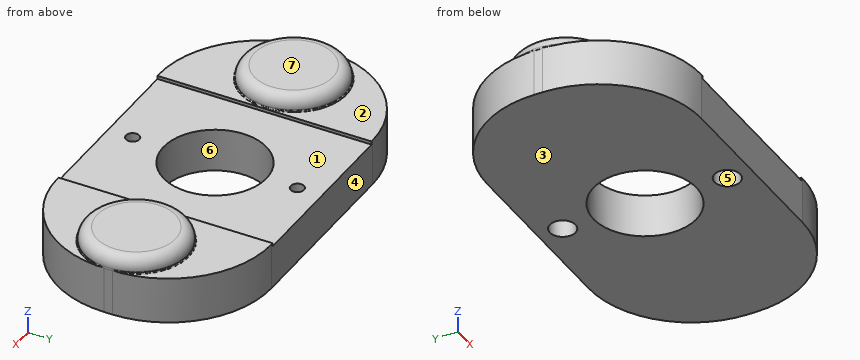
```python
from build123d import *

# Parameters (mm, degrees)
F0_R          = 1.625
F1_DEPTH      = 11.3
F2_R          = 12.5
F3_DEPTH      = 11.301
F4_R          = 9.5
F5_DEPTH      = 10.5
F6_R          = 3.125
F7_DEPTH      = 5
F8_W          = 44
F8_H          = 52
F9_DEPTH      = 0.8
F10_R         = 12.539936204
F10_R_2       = 9.5
F11_DEPTH     = 1
F12_R         = 12.54
F13_DEPTH     = 2.5
F16_T4_ANGLE  = 178.2861059353
F16_S5_R      = 25
F16_T6_DEPTH  = 17
F16_T10_ANGLE = 178.2861059353
F16_S11_R     = 25
F16_T12_DEPTH = 17
F16_T16_ANGLE = 356.5984947452
F16_S17_R     = 25
F16_T18_DEPTH = 21
F16_T22_ANGLE = 356.5984947452
F16_S23_R     = 25
F16_T24_DEPTH = 21


# Not quite as in the source:
# - a fillet or chamfer that OpenCascade refuses, or shapes differently, is made with other operations: its cross-section is extruded or revolved along the edge and cut away or added
# - a feature of the source that left no trace in its solid (it failed there, or was rolled back) is left out


with BuildPart() as f1:
    # F0 (on Top) → F1 (new body)
    with BuildSketch(Plane.XY):
        with BuildLine():
            Line((-22.5, -26), (22.5, -26))
            ThreePointArc((22.5, -26), (40.1776695297, -18.6776695297), (47.5, -1))
            Line((47.5, -1), (47.5, 1))
            ThreePointArc((47.5, 1), (40.1776695297, 18.6776695297), (22.5, 26))
            Line((22.5, 26), (-22.5, 26))
            ThreePointArc((-22.5, 26), (-40.1776695297, 18.6776695297), (-47.5, 1))
            Line((-47.5, 1), (-47.5, -1))
            ThreePointArc((-47.5, -1), (-40.1776695297, -18.6776695297), (-22.5, -26))
        make_face()
        with Locations((0, -20)):
            Circle(F0_R, mode=Mode.SUBTRACT)
        with Locations((0, 20)):
            Circle(F0_R, mode=Mode.SUBTRACT)
    extrude(amount=F1_DEPTH)

    # F2 (on face) → F3 (cut, through all)
    with BuildSketch(Plane(origin=(0, 0, 0), x_dir=(1, 0, 0), z_dir=(0, 0, -1))):
        Circle(F2_R)
    extrude(amount=-F3_DEPTH, mode=Mode.SUBTRACT)

    # F4 (on face) → F5 (cut)
    with BuildSketch(Plane.XY.offset(11.3)):
        with Locations((-35, 0)):
            Circle(F4_R)
        with Locations((35, 0)):
            Circle(F4_R)
    extrude(amount=-F5_DEPTH, mode=Mode.SUBTRACT)

    # F6 (on face) → F7 (cut)
    with BuildSketch(Plane(origin=(0, 0, 0), x_dir=(1, 0, 0), z_dir=(0, 0, -1))):
        with Locations((0, 20)):
            Circle(F6_R)
        with Locations((0, -20)):
            Circle(F6_R)
    extrude(amount=-F7_DEPTH, mode=Mode.SUBTRACT)

    # F8 (on face) → F9 (cut)
    with BuildSketch(Plane.XY.offset(11.3)):
        Rectangle(F8_W, F8_H)
    extrude(amount=-F9_DEPTH, mode=Mode.SUBTRACT)

    # F10 (on face) → F11 (join)
    with BuildSketch(Plane.XY.offset(11.3)):
        with Locations((-35, 0)):
            Circle(F10_R)
        with Locations((-35, 0)):
            Circle(F10_R_2, mode=Mode.SUBTRACT)
        with Locations((35, 0)):
            Circle(F10_R)
        with Locations((35, 0)):
            Circle(F10_R_2, mode=Mode.SUBTRACT)
    extrude(amount=F11_DEPTH)

    # F12 (on face) → F13 (join)
    with BuildSketch(Plane.XY.offset(12.3)):
        with Locations((-35, 0)):
            Circle(F12_R)
        with Locations((35, 0)):
            Circle(F12_R)
    extrude(amount=F13_DEPTH)

    # F14: fillet of radius 3 on 1 edges, made by hand

    # F14_s1 → F14_t2 (revolve, cut)
    with BuildSketch(Plane.XZ):
        with BuildLine():
            ThreePointArc((-22.46, 11.8), (-23.3386796564, 13.9213203436), (-25.46, 14.8))
            Line((-25.46, 14.8), (-22.46, 14.8))
            Line((-22.46, 14.8), (-22.46, 11.8))
        make_face()
    revolve(axis=Axis((-35, 0, 14.8), (0, 0, 1)), mode=Mode.SUBTRACT)

    # F15: fillet of radius 3 on 1 edges, made by hand

    # F15_s1 → F15_t2 (revolve, cut)
    with BuildSketch(Plane.XZ):
        with BuildLine():
            ThreePointArc((47.54, 11.8), (46.6613203436, 13.9213203436), (44.54, 14.8))
            Line((44.54, 14.8), (47.54, 14.8))
            Line((47.54, 14.8), (47.54, 11.8))
        make_face()
    revolve(axis=Axis((35, 0, 14.8), (0, 0, 1)), mode=Mode.SUBTRACT)

    # F16: fillet of radius 0.25 on 3 edges, made by hand


with BuildPart() as f16_tool2:
    # F16_s3 → F16_t4 (revolve)
    with BuildSketch(Plane.XZ):
        with BuildLine():
            ThreePointArc((-22.460063796, 11.55), (-22.3868404913, 11.3732233047), (-22.210063796, 11.3))
            Line((-22.210063796, 11.3), (-22.460063796, 11.3))
            Line((-22.460063796, 11.3), (-22.460063796, 11.55))
        make_face()
    revolve(axis=Axis((-35, 0, 11.3), (0, 0, 1)), revolution_arc=F16_T4_ANGLE)

    # F16_s5 → F16_t6 (intersect, symmetric)
    with BuildSketch(Plane.XY.offset(11.5)):
        with Locations((-22.5, 1)):
            Circle(F16_S5_R)
    extrude(amount=F16_T6_DEPTH, both=True, mode=Mode.INTERSECT)


with BuildPart() as f1_1:
    add(f1.part)

    # F16_t1: union F16_tool2
    add(f16_tool2.part)


with BuildPart() as f16_tool8:
    # F16_s9 → F16_t10 (revolve)
    with BuildSketch(Plane(origin=(-0.0313084228, 1.046333877, 0), x_dir=(0, 0, 1), z_dir=(-0.0299086337, 0.9995526367, 0))):
        with BuildLine():
            ThreePointArc((11.55, -47.5242784902), (11.3732233047, -47.5975017949), (11.3, -47.7742784902))
            Line((11.3, -47.7742784902), (11.3, -47.5242784902))
            Line((11.3, -47.5242784902), (11.55, -47.5242784902))
        make_face()
    revolve(axis=Axis((-35, 0, 11.3), (0, 0, 1)), revolution_arc=F16_T10_ANGLE)

    # F16_s11 → F16_t12 (intersect, symmetric)
    with BuildSketch(Plane.XY.offset(11.5)):
        with Locations((-22.5, -1)):
            Circle(F16_S11_R)
    extrude(amount=F16_T12_DEPTH, both=True, mode=Mode.INTERSECT)


with BuildPart() as f1_2:
    add(f1_1.part)

    # F16_t7: union F16_tool8
    add(f16_tool8.part)


with BuildPart() as f16_tool14:
    # F16_s15 → F16_t16 (revolve)
    with BuildSketch(Plane(origin=(0.0308302837, -1.0383204819, 0), x_dir=(0, 0, 1), z_dir=(0.0296793741, -0.9995594703, 0))):
        with BuildLine():
            ThreePointArc((11.55, -47.524517666), (11.3732233047, -47.5977409707), (11.3, -47.774517666))
            Line((11.3, -47.774517666), (11.3, -47.524517666))
            Line((11.3, -47.524517666), (11.55, -47.524517666))
        make_face()
    revolve(axis=Axis((35, 0, 11.3), (0, 0, 1)), revolution_arc=F16_T16_ANGLE)

    # F16_s17 → F16_t18 (intersect, symmetric)
    with BuildSketch(Plane.XY.offset(11.5)):
        with Locations((22.5, 1)):
            Circle(F16_S17_R)
    extrude(amount=F16_T18_DEPTH, both=True, mode=Mode.INTERSECT)


with BuildPart() as f1_3:
    add(f1_2.part)

    # F16_t13: union F16_tool14
    add(f16_tool14.part)


with BuildPart() as f16_tool20:
    # F16_s21 → F16_t22 (revolve)
    with BuildSketch(Plane(origin=(0.0308302837, -1.0383204819, 0), x_dir=(0, 0, 1), z_dir=(0.0296793741, -0.9995594703, 0))):
        with BuildLine():
            ThreePointArc((11.55, -47.524517666), (11.3732233047, -47.5977409707), (11.3, -47.774517666))
            Line((11.3, -47.774517666), (11.3, -47.524517666))
            Line((11.3, -47.524517666), (11.55, -47.524517666))
        make_face()
    revolve(axis=Axis((35, 0, 11.3), (0, 0, 1)), revolution_arc=F16_T22_ANGLE)

    # F16_s23 → F16_t24 (intersect, symmetric)
    with BuildSketch(Plane.XY.offset(11.5)):
        with Locations((22.5, -1)):
            Circle(F16_S23_R)
    extrude(amount=F16_T24_DEPTH, both=True, mode=Mode.INTERSECT)


with BuildPart() as f1_4:
    add(f1_3.part)

    # F16_t19: union F16_tool20
    add(f16_tool20.part)


solid = f1_4.part
```
Verification items for the finished model (mm, model axes). Face numbers are marked on the shaded views. A direction names the side the tool comes from. Give positions to 0.01 mm unless a question says otherwise; leave off trailing zeros. Order: outer loops, then holes, each group sorted by start corner. A loop starts at its lowest first (then second) coordinate and runs counter-clockwise, first axis right, second up. Notation, with made-up numbers: M 56,-23 L 106,-23 A15 ccw 106,-16 Z; hole C 49.25,39.25 d5. An arc over 180 degrees is marked long. Answer in a Markdown table with one row per item. Add a question column.
Item 1: Gauge pin test, flat ends, axial feed: pin 1 (0.6 mm diameter, centred on y = -0.5, z = 6.5, fed in from +X); pin 2 (10 mm diameter, centred on x = 8, y = 18.5, fed in from +Z); pin 3 (6 mm diameter, centred on y = 10.5, z = 6, fed in from +X); pin 4 (2.5 mm diameter, centred on x = 0, y = 20, fed in from -Z). Record the tip position at first contact, or that the pin passes through.
Item 2: Section check A-A, the plane x = 0. Enter the section's corners in (y, z) (3 decimals), and give its area (3 significant figures).
Item 3: Section check C-C, the plane x = -11.5. Enter the section's corners in (y, z).
Item 4: Mould release check, pull along X, two halves, no side actions. Record for the marked faces 6 and 7: released by +X, released by -X, zero draft, split by the parting line, or undercut.
Item 5: Scan lines: probe 1 along Y at (x, z) = (0, 3.2) (3 decimals); probe 2 along Z at (x, y) = (33, -3); probe 3 along X at (y, z) = (6.5, 7.5). Record each from-to range of solid material in increasing order. Write a range as from..to.
Item 6: Section check D-D, the plane y = 20. Enter the section's corners in (x, z) (3 decimals).
Item 7: Section check B-B, the plane z = 9.5. Enter the section's corners in (x, y) (3 decimals).
Item 8: Tool access check on the marked faces 1, 2, 3, 4 and 5. Record the directions out of +Z, -Z, +X, -X, +Y, -Y that give a thin tool (end or side, any length) a straight path to the whole face; none if there is none.
Filled sheet:
| question | item | result |
|---|---|---|
| 1 | pin 1 | stops at x = 47.5 |
| 1 | pin 2 | stops at z = 10.5 |
| 1 | pin 3 | stops at x = 46.64 |
| 1 | pin 4 | passes through |
| 2 | outline | M -26,0 L -23.125,0 L -23.125,5 L -21.625,5 L -21.625,10.5 L -26,10.5 Z; M -18.375,5 L -16.875,5 L -16.875,0 L -12.5,0 L -12.5,10.5 L -18.375,10.5 Z; M 12.5,0 L 16.875,0 L 16.875,5 L 18.375,5 L 18.375,10.5 L 12.5,10.5 Z; M 21.625,5 L 23.125,5 L 23.125,0 L 26,0 L 26,10.5 L 21.625,10.5 Z |
| 2 | area | 185 mm^2 |
| 3 | outline | M -26,0 L -4.9,0 L -4.9,10.5 L -26,10.5 Z; M 4.9,0 L 26,0 L 26,10.5 L 4.9,10.5 Z |
| 4 | face 6 | undercut |
| 4 | face 7 | zero draft |
| 5 | probe 1 | y = -26..-23.125, -16.875..-12.5, 12.5..16.875, 23.125..26 |
| 5 | probe 2 | z = 0..0.8, 12.3..14.8 |
| 5 | probe 3 | x = -46.89..-41.93, -28.07..-10.68, 10.68..28.07, 41.93..46.89 |
| 6 | outline | M -38.748,0 L -3.125,0 L -3.125,5 L -1.625,5 L -1.625,10.5 L -22,10.5 L -22,11.3 L -38.748,11.3 Z; M 1.625,5 L 3.125,5 L 3.125,0 L 38.748,0 L 38.748,11.3 L 22,11.3 L 22,10.5 L 1.625,10.5 Z |
| 7 | outline | M -47.5,-1 A25 ccw -22.5,-26 L 22.5,-26 A25 ccw 47.5,-1 L 47.5,1 A25 ccw 22.5,26 L -22.5,26 A25 ccw -47.5,1 Z; hole C -35,0 d19; hole C 0,0 d25; hole C 0,-20 d3.25; hole C 0,20 d3.25; hole C 35,0 d19 |
| 8 | face 1 | +Z, +Y, -Y |
| 8 | face 2 | +Z |
| 8 | face 3 | -Z, +X, -X, +Y, -Y |
| 8 | face 4 | +Z, -Z, +X, -X, +Y |
| 8 | face 5 | -Z |
